from build123d import *

# Parameters (mm, degrees)
F0_W     = 38.1
F0_H     = 88.9
F1_DEPTH = 254
F3_DEPTH = 38.101
F5_D     = 6.35
F6_R     = 5.08
F8_D     = 6.35
F8_DEPTH = 25.4
F8_TIP   = 1.9077324654


with BuildPart() as f1:
    # F0 (on Top) → F1 (new body, symmetric)
    with BuildSketch(Plane.XY):
        Rectangle(F0_W, F0_H)
    extrude(amount=F1_DEPTH, both=True)

    # F2 (on face) → F3 (cut, through all)
    with BuildSketch(Plane.YZ.offset(19.05)):
        Polygon((-44.45, 254), (-44.45, 212.54524919), (44.45, 254), align=None)
        Polygon((-6.8792365313, -236.4804652718), (-44.45, -254), (44.45, -254), (44.45, -212.54524919), align=None)
        Polygon((-44.45, -155.9097030042), (-44.45, -254), (-6.8792365313, -236.4804652718), align=None)
    extrude(amount=-F3_DEPTH, mode=Mode.SUBTRACT)

    # F5 (through all)
    with Locations(Plane(origin=(0, -96.2278354326, -44.8717765899), x_dir=(1, 0, 0), z_dir=(0, -0.906307787, -0.4226182617))):
        with Locations((0, -147.9167961729), (0, -186.0167961729)):
            Hole(F5_D / 2)

    # F6
    f6_edges = [f1.edges().sort_by_distance(p)[0] for p in [
        (19.05, -44.45, 28.317773),
        (-19.05, -44.45, 28.317773),
        (19.05, 44.45, 20.727375),
        (-19.05, 44.45, 20.727375),
    ]]
    fillet(f6_edges, radius=F6_R)

    # F8
    with Locations(Plane(origin=(0, -89.3485989014, 191.6086886819), x_dir=(1, 0, 0), z_dir=(0, -0.4226182617, 0.906307787))):
        with Locations((0, 113.0401226202), (0, 74.9401226202)):
            Hole(F8_D / 2, depth=F8_DEPTH)
            with Locations((0, 0, -(F8_DEPTH + F8_TIP / 2))):  # 118° drill point
                Cone(0, F8_D / 2, F8_TIP, mode=Mode.SUBTRACT)


solid = f1.part
Geometry check sheet. Reference: the model listing, model coordinates, mm. Round coordinates to 2 decimals unless told otherwise and drop trailing zeros. Loops run counter-clockwise (first coordinate to the right, second up) from the corner with the lowest first, then second, coordinate; pieces in that order, holes last.
Item 1: Mould release check, pull along Y, two halves, no side actions. Record for faces 1 (the flat face through (19.05, -1, 11)), 2 (the flat face through (0.27, -25.4, -196.76)), 3 (the cylindrical face through (0.413, -13.134, 212.939)): pulls with the +Y half, pulls with the -Y half, needs draft (parallel to the pull), parting line crosses it, or undercut.
Item 2: Thickness scan on line 1 (Z direction, x = 1.5, y = 8.5); line 2 (X direction, y = -40, z = 79); line 3 (Y direction, x = -13.5, z = -199). Record the ranges inside material, lowest first.
Item 3: Gauge pin test, flat ends, axial feed: pin 1 (2 mm diameter, centred on x = -8, y = -7, fed in from +Z); pin 2 (12 mm diameter, centred on x = 12.5, y = 21, fed in from -Z); pin 3 (8 mm diameter, centred on x = -11.5, y = 31, fed in from -Z). Record the tip position at first contact, or that the pin passes through.
Item 4: Cross-section at A-A on x = -8.5. Record the boundary of the cut face in (y, z), then the cut area to 3 significant figures.
Answer sheet:
1. face 1: needs draft
1. face 2: pulls with the -Y half
1. face 3: undercut
2. line 1: z = -229.31 to -204.37, -198.2 to -162.33, -156.16 to 237.24
2. line 2: x = -19.01 to 19.01
2. line 3: y = -24.36 to 44.45
3. pin 1: stops at z = 230.47
3. pin 2: stops at z = -226.28
3. pin 3: stops at z = -220.68
4. outline: (-44.45, -155.91) - (-6.88, -236.48) - (44.45, -212.55) - (44.45, 254) - (-44.45, 212.55) - close
4. area: 39,600 mm2
